Part model, mm, in its own coordinate system. A direction names the side the tool comes from. Coordinates: 2 decimals unless noted, no trailing zeros. Write each loop counter-clockwise with the first axis right and the second up, starting at its lowest first coordinate (ties: lowest second). Pieces come first, ordered by that corner, then holes. Notation, with made-up numbers: (-3.75, 73.25) - (22.25, 73.25) arc R10 ccw to (22.25, 92.25) - close; hole circle Ø10 at (27.5, -4.75). An arc over 180 degrees is marked (long way). Use a Markdown table: item, result.
```python
from build123d import *

# Parameters (mm, degrees)
SKIZZE1_W                        = 50
SKIZZE1_H                        = 114
AUFSATZ_LINEAR_AUSTRAGEN1_DEPTH  = 2
SKIZZE2_W                        = 46
SKIZZE2_H                        = 110
AUFSATZ_LINEAR_AUSTRAGEN2_DEPTH  = 2
SCHNITT_LINEAR_AUSTRAGEN1_REACH  = 106.213
SKIZZE3_W                        = 19.5
SKIZZE3_H                        = 33
SKIZZE4_W                        = 25.5
SKIZZE4_H                        = 33
SCHNITT_LINEAR_AUSTRAGEN2_DEPTH  = 1
SKIZZE5_R                        = 3
SCHNITT_LINEAR_AUSTRAGEN3_DEPTH  = 3.9
SCHNITT_LINEAR_AUSTRAGEN4_REACH  = 106.18
SKIZZE6_W                        = 3
SKIZZE6_H                        = 12
SKIZZE10_W                       = 9
SKIZZE10_H                       = 4
SCHNITT_LINEAR_AUSTRAGEN5_DEPTH  = 2
SKIZZE11_R                       = 2
SCHNITT_LINEAR_AUSTRAGEN6_DEPTH  = 2
SKIZZE13_R                       = 2.6
SCHNITT_LINEAR_AUSTRAGEN7_DEPTH  = 105.213135755
SKIZZE14_W                       = 7.6
SKIZZE14_H                       = 2
AUFSATZ_LINEAR_AUSTRAGEN3_DEPTH  = 8
SCHNITT_LINEAR_AUSTRAGEN8_REACH  = 120.273
SKIZZE15_R                       = 3.8033663
SKIZZE16_W                       = 25.5
SKIZZE16_H                       = 3
SCHNITT_LINEAR_AUSTRAGEN10_DEPTH = 1
SKIZZE21_W                       = 13
SKIZZE21_H                       = 13
SCHNITT_LINEAR_AUSTRAGEN11_DEPTH = 2
SCHNITT_LINEAR_AUSTRAGEN12_REACH = 106.431
SKIZZE22_R                       = 4.2
SKIZZE23_W                       = 3
SKIZZE23_H                       = 4
SCHNITT_LINEAR_AUSTRAGEN13_DEPTH = 2
SKIZZE26_W                       = 9
SKIZZE26_H                       = 4.5
SCHNITT_LINEAR_AUSTRAGEN18_DEPTH = 2


with BuildPart() as part:
    # Skizze1 → Aufsatz-Linear austragen1 (new body)
    with BuildSketch(Plane(origin=(0, 0, 0), x_dir=(0, 0, -1), z_dir=(1, 0, 0))):
        with Locations((4.873417722, -42.759493671)):
            Rectangle(SKIZZE1_W, SKIZZE1_H)
    extrude(amount=AUFSATZ_LINEAR_AUSTRAGEN1_DEPTH)

    # Skizze2 → Aufsatz-Linear austragen2 (add)
    with BuildSketch(Plane(origin=(2, 0, 0), x_dir=(0, 0, -1), z_dir=(1, 0, 0))):
        with Locations((4.873417722, -42.759493671)):
            Rectangle(SKIZZE2_W, SKIZZE2_H)
    extrude(amount=AUFSATZ_LINEAR_AUSTRAGEN2_DEPTH)

    # Skizze3 → Schnitt-Linear austragen1 (cut, up to next)
    with BuildSketch(Plane(origin=(4, 0, 0), x_dir=(0, 0, -1), z_dir=(1, 0, 0)), mode=Mode.PRIVATE) as schnitt_linear_austragen1_sk1:
        with Locations((13.123417722, -19.259493671)):
            Rectangle(SKIZZE3_W, SKIZZE3_H)
    schnitt_linear_austragen1_tool1 = extrude(schnitt_linear_austragen1_sk1.sketch, amount=-SCHNITT_LINEAR_AUSTRAGEN1_REACH, mode=Mode.PRIVATE) & part.part
    add(schnitt_linear_austragen1_tool1.solids().sort_by_distance((4, -19.259494, -13.123418))[0], mode=Mode.SUBTRACT)

    # Skizze4 → Schnitt-Linear austragen2 (cut)
    with BuildSketch(Plane(origin=(4, 0, 0), x_dir=(0, 0, -1), z_dir=(1, 0, 0))):
        with Locations((13.123417722, -19.259493671)):
            Rectangle(SKIZZE4_W, SKIZZE4_H)
    extrude(amount=-SCHNITT_LINEAR_AUSTRAGEN2_DEPTH, mode=Mode.SUBTRACT)

    # Skizze5 → Schnitt-Linear austragen3 (cut)
    with BuildSketch(Plane(origin=(4, 0, 0), x_dir=(0, 0, -1), z_dir=(1, 0, 0))):
        with BuildLine():
            ThreePointArc((9.373417722, 0.250506329), (6.498780388, -2.746873227), (3.38389492, 0))
            Line((3.38389492, 0), (3.373417722, -2.759493671))
            Line((3.373417722, -2.759493671), (9.373417722, -2.759493671))
            Line((9.373417722, -2.759493671), (9.373417722, 0.250506329))
        make_face()
        with Locations((6.373417722, 0.250506329)):
            Circle(SKIZZE5_R)
    extrude(amount=-SCHNITT_LINEAR_AUSTRAGEN3_DEPTH, mode=Mode.SUBTRACT)

    # Skizze6 → Schnitt-Linear austragen4 (cut, up to next)
    with BuildSketch(Plane(origin=(3, 0, 0), x_dir=(0, 0, -1), z_dir=(1, 0, 0)), mode=Mode.PRIVATE) as schnitt_linear_austragen4_sk1:
        with Locations((24.373417722, -19.259493671)):
            Rectangle(SKIZZE6_W, SKIZZE6_H)
    schnitt_linear_austragen4_tool1 = extrude(schnitt_linear_austragen4_sk1.sketch, amount=-SCHNITT_LINEAR_AUSTRAGEN4_REACH, mode=Mode.PRIVATE) & part.part
    add(schnitt_linear_austragen4_tool1.solids().sort_by_distance((3, -19.259494, -24.373418))[0], mode=Mode.SUBTRACT)

    # Skizze10 → Schnitt-Linear austragen5 (cut)
    with BuildSketch(Plane(origin=(4, 0, 0), x_dir=(0, 0, -1), z_dir=(1, 0, 0))):
        with Locations((13.123417722, 10.240506329)):
            Rectangle(SKIZZE10_W, SKIZZE10_H)
    extrude(amount=-SCHNITT_LINEAR_AUSTRAGEN5_DEPTH, mode=Mode.SUBTRACT)

    # Skizze11 → Schnitt-Linear austragen6 (cut)
    with BuildSketch(Plane(origin=(4, 0, 0), x_dir=(0, 0, -1), z_dir=(1, 0, 0))):
        with Locations((20.623417722, 9.740506329)):
            Circle(SKIZZE11_R)
        with Locations((5.623417722, 9.740506329)):
            Circle(SKIZZE11_R)
    extrude(amount=-SCHNITT_LINEAR_AUSTRAGEN6_DEPTH, mode=Mode.SUBTRACT)

    # Skizze13 → Schnitt-Linear austragen7 (cut, through all)
    with BuildSketch(Plane(origin=(4, 0, 0), x_dir=(0, 0, -1), z_dir=(1, 0, 0))):
        with Locations((-10.626582278, 2.240506329)):
            Circle(SKIZZE13_R)
    extrude(amount=-SCHNITT_LINEAR_AUSTRAGEN7_DEPTH, mode=Mode.SUBTRACT)

    # Skizze14 → Aufsatz-Linear austragen3 (add)
    with BuildSketch(Plane(origin=(2, 0, 0), x_dir=(0, 0, -1), z_dir=(1, 0, 0))):
        with Locations((-10.126582278, -98.759493671)):
            Rectangle(SKIZZE14_W, SKIZZE14_H)
    extrude(amount=AUFSATZ_LINEAR_AUSTRAGEN3_DEPTH)

    # Skizze15 → Schnitt-Linear austragen8 (cut, up to next)
    with BuildSketch(Plane.XZ.offset(99.759493671), mode=Mode.PRIVATE) as schnitt_linear_austragen8_sk1:
        with Locations((10, 10.126582278)):
            Circle(SKIZZE15_R)
    schnitt_linear_austragen8_tool1 = extrude(schnitt_linear_austragen8_sk1.sketch, amount=-SCHNITT_LINEAR_AUSTRAGEN8_REACH, mode=Mode.PRIVATE) & part.part
    add(schnitt_linear_austragen8_tool1.solids().sort_by_distance((10, -99.759494, 10.126582))[0], mode=Mode.SUBTRACT)

    # Skizze16 → Schnitt-Linear austragen10 (cut)
    with BuildSketch(Plane(origin=(4, 0, 0), x_dir=(0, 0, -1), z_dir=(1, 0, 0))):
        with Locations((13.123417722, -37.259493671)):
            Rectangle(SKIZZE16_W, SKIZZE16_H)
    extrude(amount=-SCHNITT_LINEAR_AUSTRAGEN10_DEPTH, mode=Mode.SUBTRACT)

    # Skizze21 → Schnitt-Linear austragen11 (cut)
    with BuildSketch(Plane(origin=(4, 0, 0), x_dir=(0, 0, -1), z_dir=(1, 0, 0))):
        with Locations((15.306102693, -84.632709468)):
            Rectangle(SKIZZE21_W, SKIZZE21_H)
    extrude(amount=-SCHNITT_LINEAR_AUSTRAGEN11_DEPTH, mode=Mode.SUBTRACT)

    # Skizze22 → Schnitt-Linear austragen12 (cut, up to next)
    with BuildSketch(Plane(origin=(2, 0, 0), x_dir=(0, 0, -1), z_dir=(1, 0, 0)), mode=Mode.PRIVATE) as schnitt_linear_austragen12_sk1:
        with Locations((15.306102693, -84.632709468)):
            Circle(SKIZZE22_R)
    schnitt_linear_austragen12_tool1 = extrude(schnitt_linear_austragen12_sk1.sketch, amount=-SCHNITT_LINEAR_AUSTRAGEN12_REACH, mode=Mode.PRIVATE) & part.part
    add(schnitt_linear_austragen12_tool1.solids().sort_by_distance((2, -84.632709, -15.306103))[0], mode=Mode.SUBTRACT)

    # Skizze23 → Schnitt-Linear austragen13 (cut)
    with BuildSketch(Plane(origin=(4, 0, 0), x_dir=(0, 0, -1), z_dir=(1, 0, 0))):
        with Locations((7.123417722, 9.740506329)):
            Rectangle(SKIZZE23_W, SKIZZE23_H)
        with Locations((19.123417722, 9.740506329)):
            Rectangle(SKIZZE23_W, SKIZZE23_H)
    extrude(amount=-SCHNITT_LINEAR_AUSTRAGEN13_DEPTH, mode=Mode.SUBTRACT)

    # Skizze26 → Schnitt-Linear austragen18 (cut)
    with BuildSketch(Plane(origin=(4, 0, 0), x_dir=(0, 0, -1), z_dir=(1, 0, 0))):
        with Locations((13.123417722, 5.990506329)):
            Rectangle(SKIZZE26_W, SKIZZE26_H)
    extrude(amount=-SCHNITT_LINEAR_AUSTRAGEN18_DEPTH, mode=Mode.SUBTRACT)


solid = part.part
```
Item 1: Which spindle directions (+Z, -Z, +X, -X, +Y, -Y) get a long thin tool onto all of the face, cutting with end or side? Do faces 1 (the face through (2, -31, -22.873)), 2 (the face through (4, -42, 1)), 3 (the face through (3, 6, -8.623)), 4 (the face through (3, -85, -21.806)), 5 (the face through (1.6, -99.759, 0.8)). Say none if no direction does.
From the geometry:
| item | result |
|---|---|
| face 1 | +X, -X |
| face 2 | +Z, -Z, +X, +Y |
| face 3 | +X, +Y |
| face 4 | +X |
| face 5 | +Z, -Z, +X, -X, -Y |
Item 2: Drill centre lines: probe 1 along Y at (x, z) = (2.5, -25.5); probe 2 along Z at (x, y) = (1.25, -1); probe 3 along Z at (x, y) = (1, -12). Where is each one in solid material? Low to high.
From the geometry:
| item | result |
|---|---|
| probe 1 | -97.76 to -25.26, -13.26 to 12.24 |
| probe 2 | -29.87 to -9.37, -3.38 to 20.13 |
| probe 3 | -29.87 to -22.87, -3.37 to 20.13 |
Item 3: Drop flat-ended pins along their axis: P1, Ø1.6, axis at x = 3, z = -18.5, coming from the +Y side; P2, Ø1.6, axis at x = 3.5, z = -12.5, coming from the +Y side; P3, Ø2, axis at x = 3.5, y = -84, coming from the -Z side; P4, Ø1.5, axis at x = 5.5, y = -7.5, coming from the -Z side. Give the stop position or say it passes through.
From the geometry:
| item | result |
|---|---|
| P1 | y = 12.24 |
| P2 | y = 3.74 |
| P3 | z = -27.87 |
| P4 | through |
Item 4: Band-saw the part on D-D, the plane z = -13.5. Give the cut face in (x, y), then the cut area to 3 significant figures.
From the geometry:
| item | result |
|---|---|
| outline | (0, -99.76) - (2, -99.76) - (2, -97.76) - (4, -97.76) - (4, -91.13) - (2, -91.13) - (2, -88.42) - (0, -88.42) - close; (0, -80.84) - (2, -80.84) - (2, -78.13) - (4, -78.13) - (4, -38.76) - (3, -38.76) - (3, -35.76) - (0, -35.76) - close; (0, -2.76) - (4, -2.76) - (4, 3.74) - (2, 3.74) - (2, 14.24) - (0, 14.24) - close |
| area | 255 mm^2 |
Item 5: Two-plate mould, pull along Z, no slides. Class faces 6 (the face through (3, 11.741, -19)), 7 (the face through (3, 12.241, -23)), 8 (the face through (3, 3.741, -13)): pulls with the +Z half, pulls with the -Z half, needs draft (parallel to the pull), parting line crosses it, or undercut.
From the geometry:
| item | result |
|---|---|
| face 6 | undercut |
| face 7 | needs draft |
| face 8 | undercut |
Item 6: Band-saw the part on A-A, the plane y = -29.5. Give the cut face in (x, z).
From the geometry:
| item | result |
|---|---|
| outline | (0, -29.87) - (2, -29.87) - (2, -27.87) - (4, -27.87) - (4, -25.87) - (3, -25.87) - (3, -22.87) - (0, -22.87) - close; (0, -3.37) - (3, -3.37) - (3, -0.37) - (4, -0.37) - (4, 18.13) - (2, 18.13) - (2, 20.13) - (0, 20.13) - close |
Item 7: Band-saw the part on B-B, the plane z = -24.5. Give the cut face in (x, y).
From the geometry:
| item | result |
|---|---|
| outline | (0, -99.76) - (2, -99.76) - (2, -97.76) - (4, -97.76) - (4, -38.76) - (3, -38.76) - (3, -25.26) - (0, -25.26) - close; (0, -13.26) - (3, -13.26) - (3, -2.76) - (4, -2.76) - (4, 12.24) - (2, 12.24) - (2, 14.24) - (0, 14.24) - close |
Item 8: Band-saw the part on C-C, the plane y = -49. Give the cut face in (x, z), then the cut area to 3 significant figures.
From the geometry:
| item | result |
|---|---|
| outline | (0, -29.87) - (2, -29.87) - (2, -27.87) - (4, -27.87) - (4, 18.13) - (2, 18.13) - (2, 20.13) - (0, 20.13) - close |
| area | 192 mm^2 |
